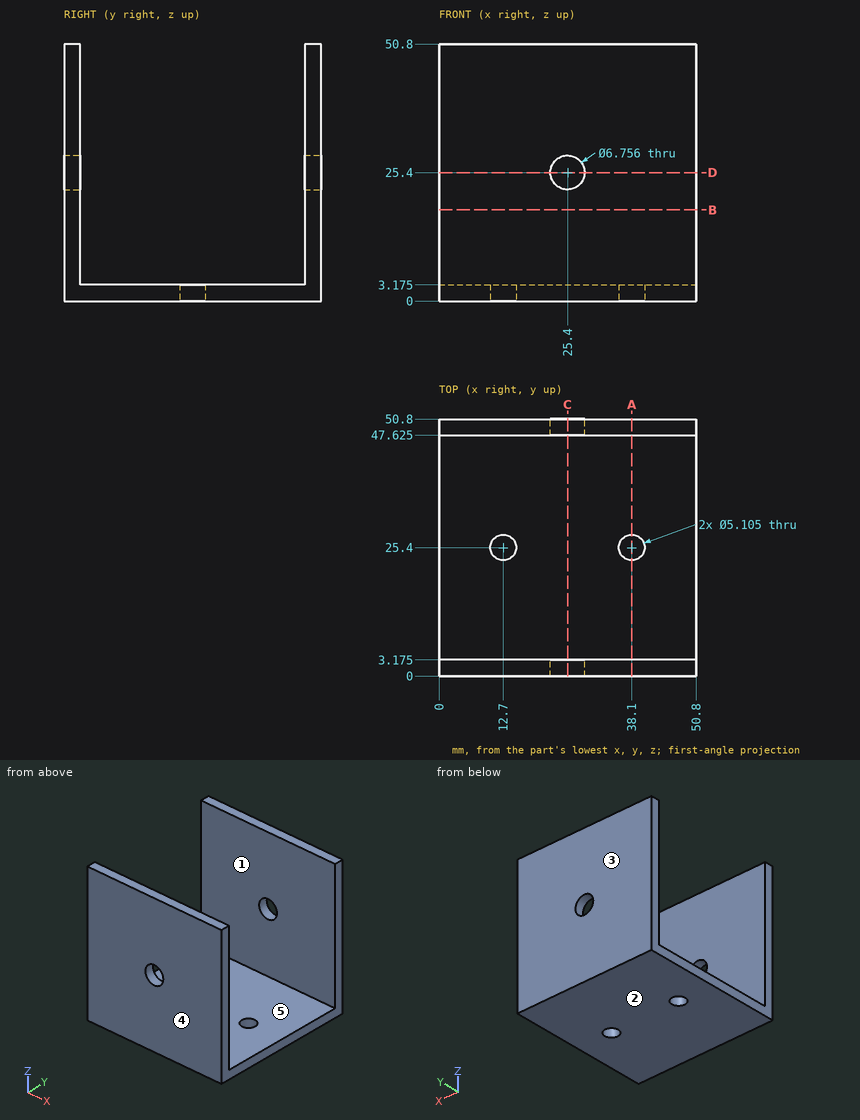
Could you check a few things on this drawing? It's one solid part, dimensions in mm from its lowest x, y, z. A direction names the side the tool comes from. Coordinates: 2 decimals unless noted, no trailing zeros. Order: outer loops, then holes, each group sorted by start corner. A loop starts at its lowest first (then second) coordinate and runs counter-clockwise, first axis right, second up. Notation, with made-up numbers: M 49,16.5 L 99,16.5 A36 ccw 99,51.5 Z; hole C -29.75,-10.5 d2. An arc over 180 degrees is marked long. Answer as a JSON object with one key per item and string values. Group by question number.
(1) If we mould it in two halves opening along Y, with no side actions, what happens to the marked faces 1, 2 and 3? For each: released by +Y, released by -Y, zero draft, split by the parting line, or undercut.
(2) For pin 1 (22 mm diameter, centred on x = 38, y = 23.5, fed in from +Z) (3 decimals), with a flat end and sliding along its axis, tell me the tip position at first contact or that it passes through.
(3) Suppose I cut it at D-D, the plane z = 25.4. Please give me the cut outline in (x, y) (1 decimal).
(4) I need wall thicknesses on probe 1 along Y at (x, z) = (38.5, 9) (1 decimal); probe 2 along Y at (x, z) = (38.1, 2.2); probe 3 along Z at (x, y) = (25, 42) (1 decimal). Which ranges of each line are inside material? Lowest first, please.
(5) Suppose I cut it at A-A, the plane x = 38.1. Please give me the cut outline in (y, z) (1 decimal).
(6) Suppose I cut it at B-B, the plane z = 18. Please give me the cut outline in (x, y) (1 decimal).
(7) Suppose I cut it at C-C, the plane x = 25.4. Please give me the cut outline in (y, z) (1 decimal), then the cut area to 3 significant figures.
(8) Which directions (+Z, -Z, +X, -X, +Y, -Y) give clear straight access to the entire face, cutting with the end or side of a thin tool? Please do the marked faces 4 and 5.
Values found:
{
 "1": {"face 1": "undercut", "face 2": "zero draft", "face 3": "released by +Y"},
 "2": {"pin 1": "stops at z = 3.175"},
 "3": {"outline": "M 0,0 L 22,0 L 22,3.2 L 0,3.2 Z; M 0,47.6 L 22,47.6 L 22,50.8 L 0,50.8 Z; M 28.8,0 L 50.8,0 L 50.8,3.2 L 28.8,3.2 Z; M 28.8,47.6 L 50.8,47.6 L 50.8,50.8 L 28.8,50.8 Z"},
 "4": {"probe 1": "y = 0 to 3.2, 47.6 to 50.8", "probe 2": "y = 0 to 22.85, 27.95 to 50.8", "probe 3": "z = 0 to 3.2"},
 "5": {"outline": "M 0,0 L 22.8,0 L 22.8,3.2 L 3.2,3.2 L 3.2,50.8 L 0,50.8 Z; M 28,0 L 50.8,0 L 50.8,50.8 L 47.6,50.8 L 47.6,3.2 L 28,3.2 Z"},
 "6": {"outline": "M 0,0 L 50.8,0 L 50.8,3.2 L 0,3.2 Z; M 0,47.6 L 50.8,47.6 L 50.8,50.8 L 0,50.8 Z"},
 "7": {"outline": "M 0,0 L 50.8,0 L 50.8,22 L 47.6,22 L 47.6,3.2 L 3.2,3.2 L 3.2,22 L 0,22 Z; M 0,28.8 L 3.2,28.8 L 3.2,50.8 L 0,50.8 Z; M 47.6,28.8 L 50.8,28.8 L 50.8,50.8 L 47.6,50.8 Z", "area": "421 mm^2"},
 "8": {"face 4": "+Z, -Z, +X, -X, -Y", "face 5": "+Z, +X, -X"}
}
